from build123d import *

# Parameters (mm, degrees)
F1_DEPTH = 40
F3_R     = 3
F4_DEPTH = 3
F5_R     = 1.5
F6_DEPTH = 12
F7_SIZE  = 3


with BuildPart() as f1:
    # F0 (on Top) → F1 (new body)
    with BuildSketch(Plane.XY):
        Polygon((0, 85.3687158704), (0, 86.5687158704), (-10, 86.5687158704), (-10, -85.9312841296), (0, -85.9312841296), (0, -84.7312841296), align=None)
        Polygon((1.2, 86.5687158704), (0, 86.5687158704), (0, 85.3687158704), align=None)
        Polygon((-10, 86.5687158704), (0, 86.5687158704), (1.2, 86.5687158704), (5.2, 86.5687158704), (7.4, 86.5687158704), (7.4, 96.5687158704), (-10, 96.5687158704), align=None)
        Polygon((0, -85.9312841296), (-10, -85.9312841296), (-10, -95.9312841296), (7.4, -95.9312841296), (7.4, -85.9312841296), (5.2, -85.9312841296), (1.2, -85.9312841296), align=None)
        Polygon((1.2, -85.9312841296), (0, -84.7312841296), (0, -85.9312841296), align=None)
        Polygon((7.4, 86.5687158704), (5.2, 86.5687158704), (7.4, 85.3687158704), align=None)
        Polygon((7.4, -84.7312841296), (5.2, -85.9312841296), (7.4, -85.9312841296), align=None)
    extrude(amount=F1_DEPTH)


with BuildPart() as f1_1:
    # F2: moved
    add(f1.part.moved(Location((0, 0, -20))))

    # F3 (on face) → F4 (cut)
    with BuildSketch(Plane.YZ):
        with Locations((0, 11.7)):
            Circle(F3_R)
        with Locations((0, -11.7)):
            Circle(F3_R)
    extrude(amount=-F4_DEPTH, mode=Mode.SUBTRACT)

    # F5 (on face) → F6 (cut)
    with BuildSketch(Plane.YZ):
        with Locations((0, 11.7)):
            Circle(F5_R)
        with Locations((0, -11.7)):
            Circle(F5_R)
    extrude(amount=-F6_DEPTH, mode=Mode.SUBTRACT)

    # F7
    f7_edges = [f1_1.edges().sort_by_distance(p)[0] for p in [
        (-1.3, -95.931284, 20),
        (-10, -95.931284, 0),
        (7.4, -95.931284, 0),
        (-1.3, -95.931284, -20),
        (7.4, 96.568716, 0),
        (-10, 96.568716, 0),
        (-1.3, 96.568716, -20),
        (-1.3, 96.568716, 20),
        (-10, 0.318716, 20),
        (-10, 0.318716, -20),
    ]]
    chamfer(f7_edges, length=F7_SIZE)


solid = f1_1.part
Design review of the part built by this model. Coordinates are the model's own, in mm. A direction names the side the tool comes from. Coordinates: 2 decimals unless noted, no trailing zeros. Write each loop counter-clockwise with the first axis right and the second up, starting at its lowest first coordinate (ties: lowest second). Pieces come first, ordered by that corner, then holes. Notation, with made-up numbers: (76, 56.5) - (107, 56.5) arc R32 ccw to (107, 83.5) - close; hole circle Ø10 at (19.25, 60). An arc over 180 degrees is marked (long way). One line per item, written item: value.
1) Add section B-B (y = 7). State the section outline as (x, z) points.
Answer sheet:
outline: (-10, -17) - (-7, -20) - (0, -20) - (0, 20) - (-7, 20) - (-10, 17) - close
2) Add section A-A (z = 0). State the section outline as (x, y) points.
Answer sheet:
outline: (-10, -92.93) - (-7, -95.93) - (4.4, -95.93) - (7.4, -92.93) - (7.4, -84.73) - (5.2, -85.93) - (1.2, -85.93) - (0, -84.73) - (0, 85.37) - (1.2, 86.57) - (5.2, 86.57) - (7.4, 85.37) - (7.4, 93.57) - (4.4, 96.57) - (-7, 96.57) - (-10, 93.57) - close
3) Insertion check: pin 1 (4 mm diameter, centred on y = -9, z = 8, fed in from +X); pin 2 (5 mm diameter, centred on y = 0, z = 11.7, fed in from +X); pin 3 (2.5 mm diameter, centred on y = 0, z = -11.7, fed in from -X). Each pin has a flat end and moves straight along its axis. Give the tip position at first contact, or say it passes through.
Answer sheet:
pin 1: stops at x = 0
pin 2: stops at x = -3
pin 3: passes through
4) To check wall thickness, follow probe 1 along Z at (x, y) = (-1.15, 0); probe 2 along Z at (x, y) = (-5.75, 0); probe 3 along X at (y, z) = (-39, 12). State the ranges of each line that lie inside material, in increasing order.
Answer sheet:
probe 1: z = -20 to -14.7, -8.7 to 8.7, 14.7 to 20
probe 2: z = -20 to -13.2, -10.2 to 10.2, 13.2 to 20
probe 3: x = -10 to 0
5) For faces 1 (the face through (-1.479, -0.391, -8.726)), 2 (the face through (0, -1, 0)), 3 (the face through (0.3, 95.09, 18.48)), list the 3-axis set-ups (+Z, -Z, +X, -X, +Y, -Y) from which the entire face can be reached by the end or side of a thin tool; tool diameter is ignored.
Answer sheet:
face 1: +X
face 2: +Z, -Z, +X
face 3: +Z, +X, -X, +Y
6) Mouldability with a two-part tool opening along Z and no side actions: class faces 4 (the face through (-7.906, 94.517, 18.146)), 5 (the face through (-3, 1, -10)), 6 (the face through (-1, 96.569, 0)) as +Z half, -Z half, draft (parallel to the pull), parting line (faces both ways), or undercut.
Answer sheet:
face 4: +Z half
face 5: undercut
face 6: draft
